The figure shows three views and two pictorial views of one solid part (mm, origin at its lowest corner). Answer the questions. Round coordinates to 2 decimals unless told otherwise and drop trailing zeros. Order: outer loops, then holes, each group sorted by start corner. A loop starts at its lowest first (then second) coordinate and runs counter-clockwise, first axis right, second up. Notation, with made-up numbers: (73.25, 14.25) - (94.25, 14.25) arc R29 cw to (94.25, 45.25) - close; hole circle Ø1 at (42.5, 63). An arc over 180 degrees is marked (long way). Write item = value, one per line.
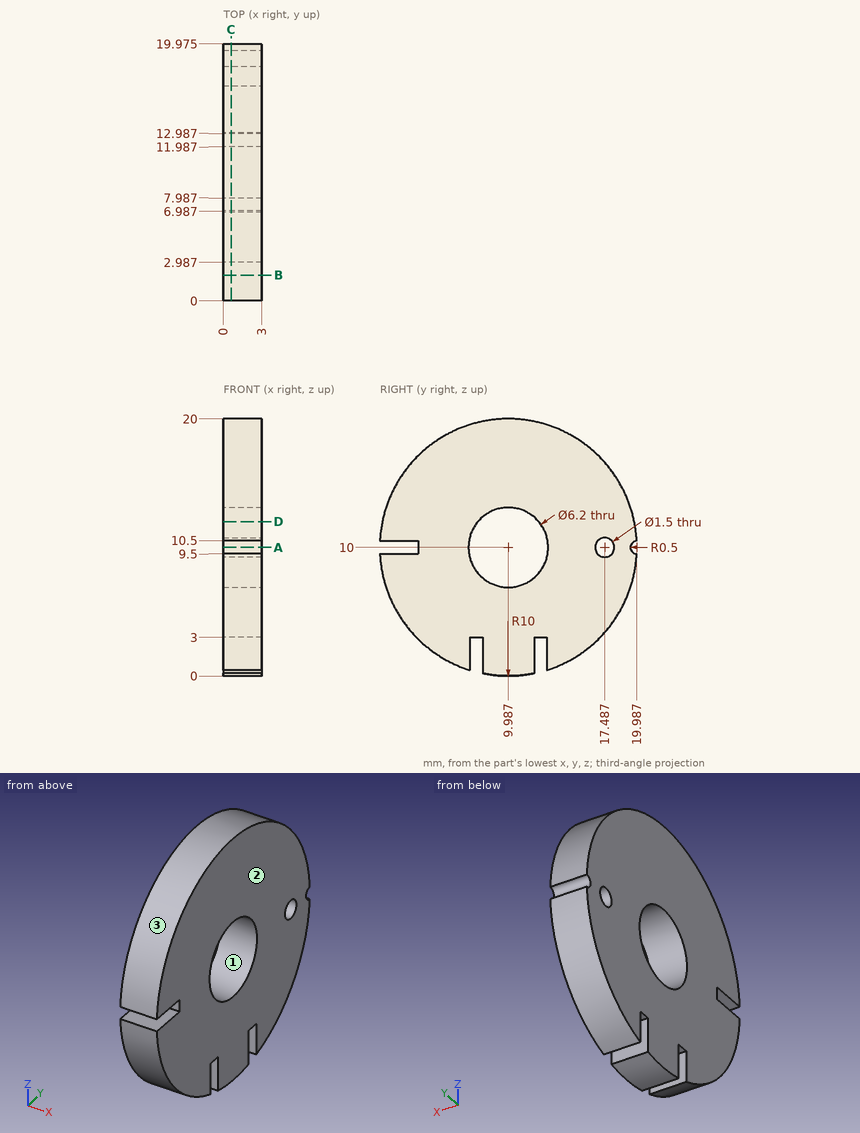
Q1. Section C-C on x = 0.6 is taken. Count the separate pieces of the cut face and the enclosed holes in it.
Model answer:
separate_pieces = 1
enclosed_holes = 2
Q2. Section D-D on z = 12 is taken. Determine the outline of the cut face in (x, y) (1 decimal).
Model answer:
outline = (0, 0.2) - (3, 0.2) - (3, 7.6) - (0, 7.6) - close; (0, 12.4) - (3, 12.4) - (3, 19.8) - (0, 19.8) - close
Q3. Section B-B on y = 2 is taken. Determine the outline of the cut face in (x, z), then the cut area to 3 significant figures.
Model answer:
outline = (0, 3.98) - (3, 3.98) - (3, 9.5) - (0, 9.5) - close; (0, 10.5) - (3, 10.5) - (3, 16.02) - (0, 16.02) - close
area = 33.1 mm^2
Q4. Section A-A on z = 10 is taken. Determine the outline of the cut face in (x, y).
Model answer:
outline = (0, 2.99) - (3, 2.99) - (3, 6.89) - (0, 6.89) - close; (0, 13.09) - (3, 13.09) - (3, 16.74) - (0, 16.74) - close; (0, 18.24) - (3, 18.24) - (3, 19.49) - (0, 19.49) - close
Q5. Find the intervals of material crossed by line 1 (Z direction, x = 0.85, y = 9); line 2 (Z direction, x = 0.55, y = 17.25) (1 decimal); line 3 (Y direction, x = 1.7, z = 12) (1 decimal), in increasing order. Write a range as from..to.
Model answer:
line_1 = 0.05..7.06, 12.94..19.95
line_2 = 3.1..9.3, 10.7..16.9
line_3 = 0.2..7.6, 12.4..19.8
Q6. Flat-ended cylindrical pins translate along their axes: P1, Ø0.9, axis at x = 1, y = 1, coming from the -Z side (1 decimal); P2, Ø1.4, axis at x = 2, z = 1, coming from the +Y side (1 decimal); P3, Ø3.5, axis at y = 9.99, z = 10, coming from the -X side; P4, Ø0.5, axis at x = 1.5, y = 7.5, coming from the -Z side. Find the tip coordinate at first contact, or state that the pin passes through.
Model answer:
P1 = 4.8
P2 = 15.6
P3 = through
P4 = 3
Q7. Determine the mould class of the marked faces 1, 2 and 3 for opening direction Y: released by +Y, released by -Y, zero draft, split by the parting line, or undercut.
Model answer:
face_1 = undercut
face_2 = zero draft
face_3 = split by the parting line
